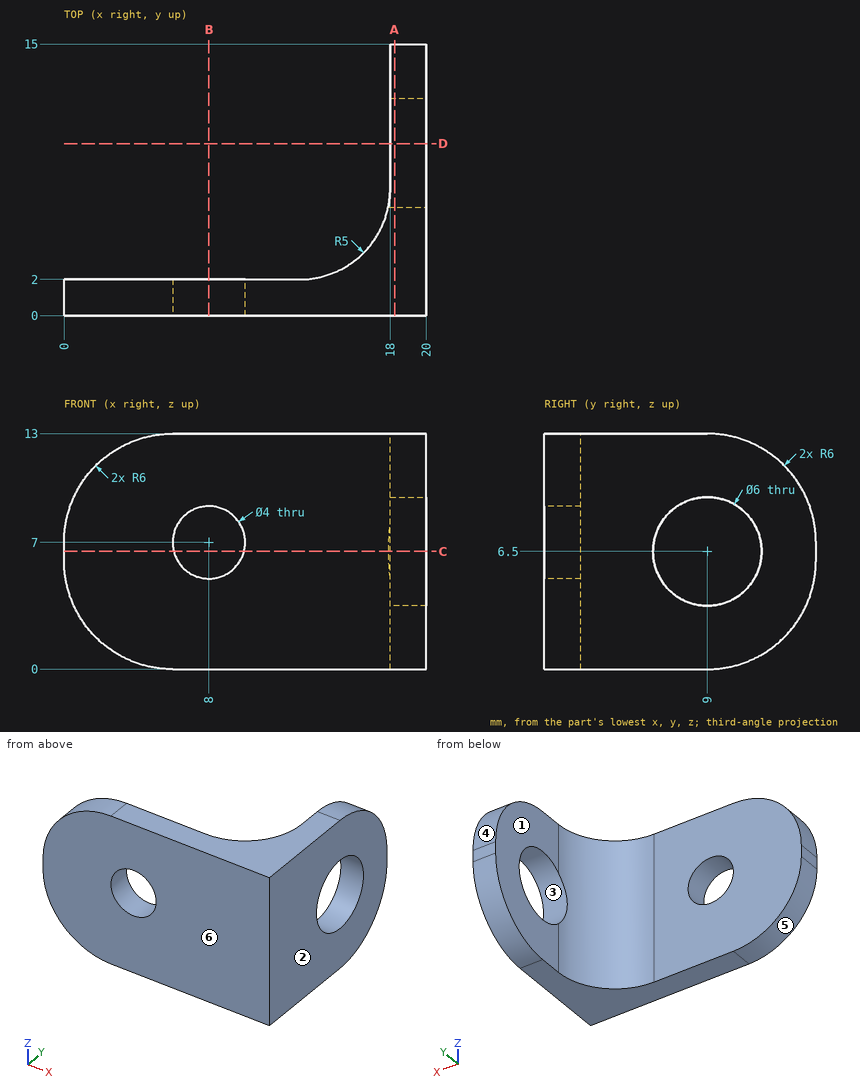
Print and shaded views of the part. All mm, measured from the part's lowest x, y and z. A direction names the side the tool comes from. Give positions to 0.01 mm unless a question says otherwise; leave off trailing zeros. Loops run counter-clockwise (first coordinate to the right, second up) from the corner with the lowest first, then second, coordinate; pieces in that order, holes last. Notation, with made-up numbers: (59.25, 66) - (90.25, 66) arc R8 ccw to (90.25, 81) - close; hole circle Ø4 at (85, -1.5). An arc over 180 degrees is marked (long way). Use a Markdown table: item, result.
(1) Band-saw the part on C-C (z = 6.5). Give the cut face in (x, y), and give its area (3 significant figures).
Taken from the geometry:
| item | result |
|---|---|
| outline | (0, 0) - (6.06, 0) - (6.06, 2) - (0, 2) - close; (9.94, 0) - (20, 0) - (20, 6) - (17.9, 6) arc R5 cw to (13, 2) - (9.94, 2) - close; (18, 12) - (20, 12) - (20, 15) - (18, 15) - close |
| area | 51.6 mm2 |
(2) Which spindle directions (+Z, -Z, +X, -X, +Y, -Y) get a long thin tool onto all of the face, cutting with end or side? Do the marked faces 1 and 2. Say none if no direction does.
Taken from the geometry:
| item | result |
|---|---|
| face 1 | +Z, -Z, -X, +Y |
| face 2 | +Z, -Z, +X, +Y, -Y |
(3) Wall check: line 1 along Z through (x, y) = (19.45, 9); line 2 along Z through (x, y) = (8, 0.5); line 3 along Y through (x, z) = (19.5, 6.5). Give the ranges that are in metal, low to high.
Taken from the geometry:
| item | result |
|---|---|
| line 1 | 0 to 3.5, 9.5 to 13 |
| line 2 | 0 to 5, 9 to 13 |
| line 3 | 0 to 6, 12 to 15 |
(4) Band-saw the part on A-A (x = 18.25). Give the cut face in (y, z), and give its area (3 significant figures).
Taken from the geometry:
| item | result |
|---|---|
| outline | (0, 0) - (9, 0) arc R6 ccw to (15, 6) - (15, 7) arc R6 ccw to (9, 13) - (0, 13) - close; hole circle Ø6 at (9, 6.5) |
| area | 151 mm2 |
(5) Pull direction Y, two halves, no side cores. Call the marked faces 3, 4, 5 and 6: +Y half, -Y half, draft (parallel to the pull), parting line (faces both ways), or undercut.
Taken from the geometry:
| item | result |
|---|---|
| face 3 | undercut |
| face 4 | +Y half |
| face 5 | draft |
| face 6 | -Y half |
(6) Band-saw the part on D-D (y = 9.5). Give the cut face in (x, z), and give its area (3 significant figures).
Taken from the geometry:
| item | result |
|---|---|
| outline | (18, 0.02) - (20, 0.02) - (20, 3.54) - (18, 3.54) - close; (18, 9.46) - (20, 9.46) - (20, 12.98) - (18, 12.98) - close |
| area | 14.1 mm2 |
(7) Drop flat-ended pins along their axis: pin 1 Ø2 at (y, z) = (4.5, 9.5) entering from -X; pin 2 Ø6.5 at (x, z) = (8, 7) entering from +Y; pin 3 Ø3.5 at (y, z) = (9, 6.5) entering from -X. Give the stop position or say it passes through.
Taken from the geometry:
| item | result |
|---|---|
| pin 1 | x = 16.57 |
| pin 2 | y = 2 |
| pin 3 | through |
(8) Band-saw the part on B-B (x = 8). Give the cut face in (y, z), and give its area (3 significant figures).
Taken from the geometry:
| item | result |
|---|---|
| outline | (0, 0) - (2, 0) - (2, 5) - (0, 5) - close; (0, 9) - (2, 9) - (2, 13) - (0, 13) - close |
| area | 18.0 mm2 |
